from build123d import *

# Parameters (mm, degrees)
EXTRUDE_1_DEPTH     = 6
CUT_EXTRUDE_START   = -1
SKETCH_4_W          = 37.365757144
SKETCH_4_H          = 18.186872946
SKETCH_4_R          = 5
CUT_EXTRUDE_1_DEPTH = 1
CHAMFER_1_SIZE      = 0.5


with BuildPart() as part:
    # 草图1 → 凸台-拉伸1 (new body)
    with BuildSketch(Plane(origin=(0, 0, 0), x_dir=(1, 0, 0), z_dir=(0, 1, 0))):
        with BuildLine():
            Line((0, 5), (23, 5))
            ThreePointArc((23, 5), (28, 0), (23, -5))
            Line((23, -5), (0, -5))
            ThreePointArc((0, -5), (-5, 0), (0, 5))
        make_face()
    extrude(amount=EXTRUDE_1_DEPTH)

    # 草图2 → 切除-旋转1 (revolve, cut)
    with BuildSketch(Plane.XY, mode=Mode.PRIVATE) as cut_revolve_1_sk:
        Polygon((0, 0), (-3.75, 0), (-3.75, 3.5), (-2.075, 3.5), (-2.075, 6), (0, 6), align=None)
    revolve(cut_revolve_1_sk.sketch.rotate(Axis((0, 6, 0), (0, -1, 0)), 270), axis=Axis((0, 6, 0), (0, -1, 0)), mode=Mode.SUBTRACT)

    # 草图3 → 切除-旋转2 (revolve, cut)
    with BuildSketch(Plane.XY, mode=Mode.PRIVATE) as cut_revolve_2_sk:
        Polygon((23, 0), (19.25, 0), (19.25, 3.5), (20.925, 3.5), (20.925, 6), (23, 6), align=None)
    revolve(cut_revolve_2_sk.sketch.rotate(Axis((23, 0, 0), (0, 1, 0)), 270), axis=Axis((23, 0, 0), (0, 1, 0)), mode=Mode.SUBTRACT)

    # 草图4 → 切除-拉伸1 (cut)
    with BuildSketch(Plane(origin=(0, 6, 0), x_dir=(1, 0, 0), z_dir=(0, 1, 0)).offset(CUT_EXTRUDE_START)):
        with Locations((11.904152732, 0.202076366)):
            Rectangle(SKETCH_4_W, SKETCH_4_H)
        with Locations(Location((0, 0, 0), (0, 0, 270))):
            Circle(SKETCH_4_R, mode=Mode.SUBTRACT)
        with Locations(Location((23, 0, 0), (0, 0, 270))):
            Circle(SKETCH_4_R, mode=Mode.SUBTRACT)
    extrude(amount=CUT_EXTRUDE_1_DEPTH, mode=Mode.SUBTRACT)

    # 倒角1
    chamfer_1_edges = [part.edges().sort_by_distance(p)[0] for p in [
        (23, 6, 5),
        (0, 6, -5),
        (11.5, 0, -5),
        (28, 0, 0),
        (11.5, 0, 5),
        (-5, 0, 0),
    ]]
    chamfer(chamfer_1_edges, length=CHAMFER_1_SIZE)


solid = part.part
Model file for the job. Use its own axes, mm. A direction names the side the tool comes from. Give positions to 0.01 mm unless a question says otherwise; leave off trailing zeros. Order: outer loops, then holes, each group sorted by start corner. A loop starts at its lowest first (then second) coordinate and runs counter-clockwise, first axis right, second up. Notation, with made-up numbers: M -17.75,87 L 7.25,87 A13 cw 7.25,104 Z; hole C -30,-19 d5. An arc over 180 degrees is marked long. Put each result on its own line as item: value. Start each with the question number.
(1) Tool access for faces 5 (the face through (2, 3.5, 2)), 6 (the face through (1.26, 4.77, -1.65)): list every direction of +Z, -Z, +X, -X, +Y, -Y with a clear straight run to the whole face (end or side of a thin tool).
(2) Band-saw the part on D-D on y = 2.9. Give the cut face in (x, z), then the cut area to 3 significant figures.
(3) Band-saw the part on C-C on x = 10.5. Give the cut face in (y, z).
(4) Band-saw the part on B-B on y = 4.4. Give the cut face in (x, z) (3 decimals), then the cut area to 3 significant figures.
(5) Pin check, flat tips, straight feed: pin 1 Ø5 at (x, z) = (0, 0) entering from -Y; pin 2 Ø2 at (y, z) = (2, -3.5) entering from -X; pin 3 Ø1 at (y, z) = (5, -3.5) entering from +X. Stop position of each tip, or through.
(6) Band-saw the part on A-A on z = 0. Count the separate pieces of the cut face and the enclosed holes in it, then the cut area to 3 significant figures.
(7) Pull direction X, two halves, no side cores. Call faces 1 (the face through (27.634, 0.135, -0.102)), 2 (the face through (12, 0, 0)), 3 (the face through (20.943, 4.768, 0.27)), 4 (the face through (-4.634, 0.135, 0.102)): released by +X, released by -X, zero draft, split by the parting line, or undercut.
(8) Drill centre lines: L1, parallel to X at y = 5.5, z = 0 (3 decimals); L2, parallel to X at y = 4.7, z = 0 (3 decimals); L3, parallel to X at y = 0.95, z = 0. Where is each one in solid material? Low to high. Write a range as [from, to].
Results below:
1. face 5: -Y
1. face 6: +Y, -Y
2. outline: M 0,-5 L 23,-5 A5 ccw 23,5 L 0,5 A5 ccw Z; hole C 0,0 d7.5; hole C 23,0 d7.5
2. area: 220 mm2
3. outline: M 0,-4.5 L 0.5,-5 L 5,-5 L 5,5 L 0.5,5 L 0,4.5 Z
4. outline: M 0,-5 L 23,-5 A5 ccw 23,5 L 0,5 A5 ccw Z; hole C 0,0 d4.15; hole C 23,0 d4.15
4. area: 281 mm2
5. pin 1: stops at y = 3.5
5. pin 2: stops at x = -4.33
5. pin 3: stops at x = 27
6. separate pieces: 3
6. enclosed holes: 0
6. area: 111 mm2
7. face 1: released by +X
7. face 2: zero draft
7. face 3: undercut
7. face 4: released by -X
8. L1: x = [-5, -2.075], [2.075, 5], [18, 20.925], [25.075, 28]
8. L2: x = [-5, -2.075], [2.075, 20.925], [25.075, 28]
8. L3: x = [-5, -3.75], [3.75, 19.25], [26.75, 28]
